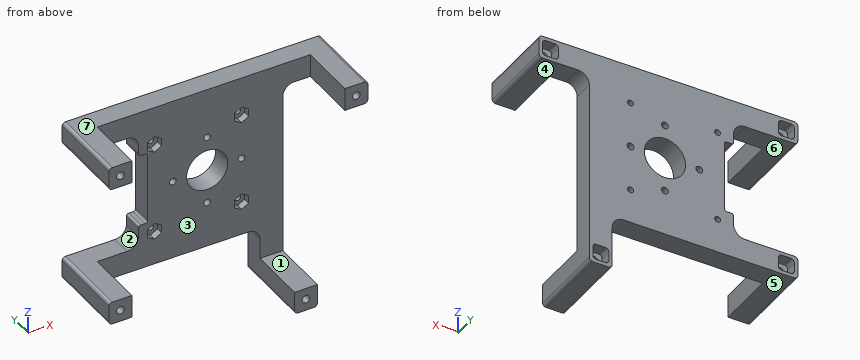
from build123d import *

# Parameters (mm, degrees)
BOSS_EXTRUDE1_DEPTH = 9
CUT_EXTRUDE1_REACH  = 11
SKETCH2_R           = 9
SKETCH2_R_2         = 1.5
CUT_EXTRUDE2_REACH  = 11
SKETCH3_R           = 1.3
SKETCH4_W           = 10
SKETCH4_H           = 10
BOSS_EXTRUDE2_DEPTH = 25.7
SKETCH5_W           = 10
SKETCH5_H           = 10
BOSS_EXTRUDE3_DEPTH = 25.7
SKETCH6_W           = 10
SKETCH6_H           = 10
BOSS_EXTRUDE4_DEPTH = 25.7
SKETCH7_W           = 10
SKETCH7_H           = 10
BOSS_EXTRUDE5_DEPTH = 25.7
SKETCH8_W           = 7
SKETCH8_H           = 7
CUT_EXTRUDE3_DEPTH  = 5
CUT_EXTRUDE4_REACH  = 31.7
SKETCH9_R           = 1.7
FILLET1_R           = 1.5
FILLET2_R           = 5
CUT_EXTRUDE7_DEPTH  = 3
FILLET3_R           = 1


with BuildPart() as part:
    # Sketch1 → Boss-Extrude1 (new body)
    with BuildSketch(Plane(origin=(0, 0, 0), x_dir=(1, 0, 0), z_dir=(0, 1, 0))):
        Polygon((-30, -27), (-30, -17), (-26, -17), (-26, 15), (-30, 15), (-30, 25), (-58, 25), (-58, 35), (23, 35), (23, 59), (33, 59), (33, 35), (33, -27), (55, -27), (55, -37), (33, -37), (-26, -37), (-58, -37), (-58, -27), align=None)
    extrude(amount=BOSS_EXTRUDE1_DEPTH)

    # Sketch2 → Cut-Extrude1 (cut, up to next)
    with BuildSketch(Plane(origin=(0, 9, 0), x_dir=(1, 0, 0), z_dir=(0, 1, 0)), mode=Mode.PRIVATE) as cut_extrude1_sk1:
        Circle(SKETCH2_R)
    cut_extrude1_tool1 = extrude(cut_extrude1_sk1.sketch, amount=-CUT_EXTRUDE1_REACH, mode=Mode.PRIVATE) & part.part
    add(cut_extrude1_tool1.solids().sort_by_distance((0, 9, 0))[0], mode=Mode.SUBTRACT)
    # Sketch2 → Cut-Extrude1 (cut, up to next)
    with BuildSketch(Plane(origin=(0, 9, 0), x_dir=(1, 0, 0), z_dir=(0, 1, 0)), mode=Mode.PRIVATE) as cut_extrude1_sk2:
        with Locations((0, 15)):
            Circle(SKETCH2_R_2)
    cut_extrude1_tool2 = extrude(cut_extrude1_sk2.sketch, amount=-CUT_EXTRUDE1_REACH, mode=Mode.PRIVATE) & part.part
    add(cut_extrude1_tool2.solids().sort_by_distance((0, 9, -15))[0], mode=Mode.SUBTRACT)
    # Sketch2 → Cut-Extrude1 (cut, up to next)
    with BuildSketch(Plane(origin=(0, 9, 0), x_dir=(1, 0, 0), z_dir=(0, 1, 0)), mode=Mode.PRIVATE) as cut_extrude1_sk3:
        with Locations((15, 0)):
            Circle(SKETCH2_R_2)
    cut_extrude1_tool3 = extrude(cut_extrude1_sk3.sketch, amount=-CUT_EXTRUDE1_REACH, mode=Mode.PRIVATE) & part.part
    add(cut_extrude1_tool3.solids().sort_by_distance((15, 9, 0))[0], mode=Mode.SUBTRACT)
    # Sketch2 → Cut-Extrude1 (cut, up to next)
    with BuildSketch(Plane(origin=(0, 9, 0), x_dir=(1, 0, 0), z_dir=(0, 1, 0)), mode=Mode.PRIVATE) as cut_extrude1_sk4:
        with Locations((0, -15)):
            Circle(SKETCH2_R_2)
    cut_extrude1_tool4 = extrude(cut_extrude1_sk4.sketch, amount=-CUT_EXTRUDE1_REACH, mode=Mode.PRIVATE) & part.part
    add(cut_extrude1_tool4.solids().sort_by_distance((0, 9, 15))[0], mode=Mode.SUBTRACT)
    # Sketch2 → Cut-Extrude1 (cut, up to next)
    with BuildSketch(Plane(origin=(0, 9, 0), x_dir=(1, 0, 0), z_dir=(0, 1, 0)), mode=Mode.PRIVATE) as cut_extrude1_sk5:
        with Locations((-15, 0)):
            Circle(SKETCH2_R_2)
    cut_extrude1_tool5 = extrude(cut_extrude1_sk5.sketch, amount=-CUT_EXTRUDE1_REACH, mode=Mode.PRIVATE) & part.part
    add(cut_extrude1_tool5.solids().sort_by_distance((-15, 9, 0))[0], mode=Mode.SUBTRACT)

    # Sketch3 → Cut-Extrude2 (cut, up to next)
    with BuildSketch(Plane(origin=(0, 9, 0), x_dir=(1, 0, 0), z_dir=(0, 1, 0)), mode=Mode.PRIVATE) as cut_extrude2_sk1:
        with Locations((-23, 20)):
            Circle(SKETCH3_R)
    cut_extrude2_tool1 = extrude(cut_extrude2_sk1.sketch, amount=-CUT_EXTRUDE2_REACH, mode=Mode.PRIVATE) & part.part
    add(cut_extrude2_tool1.solids().sort_by_distance((-23, 9, -20))[0], mode=Mode.SUBTRACT)
    # Sketch3 → Cut-Extrude2 (cut, up to next)
    with BuildSketch(Plane(origin=(0, 9, 0), x_dir=(1, 0, 0), z_dir=(0, 1, 0)), mode=Mode.PRIVATE) as cut_extrude2_sk2:
        with Locations((-23, -20)):
            Circle(SKETCH3_R)
    cut_extrude2_tool2 = extrude(cut_extrude2_sk2.sketch, amount=-CUT_EXTRUDE2_REACH, mode=Mode.PRIVATE) & part.part
    add(cut_extrude2_tool2.solids().sort_by_distance((-23, 9, 20))[0], mode=Mode.SUBTRACT)
    # Sketch3 → Cut-Extrude2 (cut, up to next)
    with BuildSketch(Plane(origin=(0, 9, 0), x_dir=(1, 0, 0), z_dir=(0, 1, 0)), mode=Mode.PRIVATE) as cut_extrude2_sk3:
        with Locations((15, 20)):
            Circle(SKETCH3_R)
    cut_extrude2_tool3 = extrude(cut_extrude2_sk3.sketch, amount=-CUT_EXTRUDE2_REACH, mode=Mode.PRIVATE) & part.part
    add(cut_extrude2_tool3.solids().sort_by_distance((15, 9, -20))[0], mode=Mode.SUBTRACT)
    # Sketch3 → Cut-Extrude2 (cut, up to next)
    with BuildSketch(Plane(origin=(0, 9, 0), x_dir=(1, 0, 0), z_dir=(0, 1, 0)), mode=Mode.PRIVATE) as cut_extrude2_sk4:
        with Locations((15, -20)):
            Circle(SKETCH3_R)
    cut_extrude2_tool4 = extrude(cut_extrude2_sk4.sketch, amount=-CUT_EXTRUDE2_REACH, mode=Mode.PRIVATE) & part.part
    add(cut_extrude2_tool4.solids().sort_by_distance((15, 9, 20))[0], mode=Mode.SUBTRACT)

    # Sketch4 → Boss-Extrude2 (add)
    with BuildSketch(Plane.XZ):
        with Locations((-53, -30)):
            Rectangle(SKETCH4_W, SKETCH4_H)
    extrude(amount=BOSS_EXTRUDE2_DEPTH)

    # Sketch5 → Boss-Extrude3 (add)
    with BuildSketch(Plane.XZ):
        with Locations((-53, 32)):
            Rectangle(SKETCH5_W, SKETCH5_H)
    extrude(amount=BOSS_EXTRUDE3_DEPTH)

    # Sketch6 → Boss-Extrude4 (add)
    with BuildSketch(Plane.XZ):
        with Locations((28, -54)):
            Rectangle(SKETCH6_W, SKETCH6_H)
    extrude(amount=BOSS_EXTRUDE4_DEPTH)

    # Sketch7 → Boss-Extrude5 (add)
    with BuildSketch(Plane.XZ):
        with Locations((50, 32)):
            Rectangle(SKETCH7_W, SKETCH7_H)
    extrude(amount=BOSS_EXTRUDE5_DEPTH)

    # Sketch8 → Cut-Extrude3 (cut)
    with BuildSketch(Plane(origin=(0, 9, 0), x_dir=(1, 0, 0), z_dir=(0, 1, 0))):
        with Locations((-53, 30)):
            Rectangle(SKETCH8_W, SKETCH8_H)
        with Locations((-53, -32)):
            Rectangle(SKETCH8_W, SKETCH8_H)
        with Locations((50, -32)):
            Rectangle(SKETCH8_W, SKETCH8_H)
        with Locations((28, 54)):
            Rectangle(SKETCH8_W, SKETCH8_H)
    extrude(amount=-CUT_EXTRUDE3_DEPTH, mode=Mode.SUBTRACT)

    # Sketch9 → Cut-Extrude4 (cut, up to next)
    with BuildSketch(Plane(origin=(0, 4, 0), x_dir=(1, 0, 0), z_dir=(0, 1, 0)), mode=Mode.PRIVATE) as cut_extrude4_sk1:
        with Locations((-53, 30)):
            Circle(SKETCH9_R)
    cut_extrude4_tool1 = extrude(cut_extrude4_sk1.sketch, amount=-CUT_EXTRUDE4_REACH, mode=Mode.PRIVATE) & part.part
    add(cut_extrude4_tool1.solids().sort_by_distance((-53, 4, -30))[0], mode=Mode.SUBTRACT)
    # Sketch9 → Cut-Extrude4 (cut, up to next)
    with BuildSketch(Plane(origin=(0, 4, 0), x_dir=(1, 0, 0), z_dir=(0, 1, 0)), mode=Mode.PRIVATE) as cut_extrude4_sk2:
        with Locations((28, 54)):
            Circle(SKETCH9_R)
    cut_extrude4_tool2 = extrude(cut_extrude4_sk2.sketch, amount=-CUT_EXTRUDE4_REACH, mode=Mode.PRIVATE) & part.part
    add(cut_extrude4_tool2.solids().sort_by_distance((28, 4, -54))[0], mode=Mode.SUBTRACT)
    # Sketch9 → Cut-Extrude4 (cut, up to next)
    with BuildSketch(Plane(origin=(0, 4, 0), x_dir=(1, 0, 0), z_dir=(0, 1, 0)), mode=Mode.PRIVATE) as cut_extrude4_sk3:
        with Locations((50, -32)):
            Circle(SKETCH9_R)
    cut_extrude4_tool3 = extrude(cut_extrude4_sk3.sketch, amount=-CUT_EXTRUDE4_REACH, mode=Mode.PRIVATE) & part.part
    add(cut_extrude4_tool3.solids().sort_by_distance((50, 4, 32))[0], mode=Mode.SUBTRACT)
    # Sketch9 → Cut-Extrude4 (cut, up to next)
    with BuildSketch(Plane(origin=(0, 4, 0), x_dir=(1, 0, 0), z_dir=(0, 1, 0)), mode=Mode.PRIVATE) as cut_extrude4_sk4:
        with Locations((-53, -32)):
            Circle(SKETCH9_R)
    cut_extrude4_tool4 = extrude(cut_extrude4_sk4.sketch, amount=-CUT_EXTRUDE4_REACH, mode=Mode.PRIVATE) & part.part
    add(cut_extrude4_tool4.solids().sort_by_distance((-53, 4, 32))[0], mode=Mode.SUBTRACT)

    # Fillet1
    fillet1_edges = [part.edges().sort_by_distance(p)[0] for p in [
        (24.5, 6.5, -57.5),
        (24.5, 6.5, -50.5),
        (31.5, 6.5, -50.5),
        (31.5, 6.5, -57.5),
        (46.5, 6.5, 28.5),
        (46.5, 6.5, 35.5),
        (53.5, 6.5, 35.5),
        (53.5, 6.5, 28.5),
        (-56.5, 6.5, 28.5),
        (-56.5, 6.5, 35.5),
        (-49.5, 6.5, 35.5),
        (-49.5, 6.5, 28.5),
        (-49.5, 6.5, -26.5),
        (-49.5, 6.5, -33.5),
        (-56.5, 6.5, -33.5),
        (-56.5, 6.5, -26.5),
        (-58, -8.35, -35),
        (23, -8.35, -59),
        (33, -8.35, -59),
        (55, -8.35, 27),
        (55, -8.35, 37),
        (-58, -8.35, 37),
        (-58, -8.35, 27),
        (-58, -8.35, -25),
    ]]
    fillet(fillet1_edges, radius=FILLET1_R)

    # Fillet2
    fillet2_edges = [part.edges().sort_by_distance(p)[0] for p in [
        (23, 4.5, -35),
        (33, 4.5, 27),
        (-30, 4.5, 27),
        (-30, 4.5, -25),
    ]]
    fillet(fillet2_edges, radius=FILLET2_R)

    # Sketch12 → Cut-Extrude7 (cut)
    with BuildSketch(Plane.XZ):
        Polygon((-19.9, 18.210214166), (-19.9, 21.789785834), (-23, 23.579571669), (-26.1, 21.789785834), (-26.1, 18.210214166), (-23, 16.420428331), align=None)
        Polygon((18.1, 21.789785834), (15, 23.579571669), (11.9, 21.789785834), (11.9, 18.210214166), (15, 16.420428331), (18.1, 18.210214166), align=None)
        Polygon((18.1, -18.210214166), (15, -16.420428331), (11.9, -18.210214166), (11.9, -21.789785834), (15, -23.579571669), (18.1, -21.789785834), align=None)
        Polygon((-19.9, -18.210214166), (-23, -16.420428331), (-26.1, -18.210214166), (-26.1, -21.789785834), (-23, -23.579571669), (-19.9, -21.789785834), align=None)
    extrude(amount=-CUT_EXTRUDE7_DEPTH, mode=Mode.SUBTRACT)

    # Fillet3
    fillet3_edges = [part.edges().sort_by_distance(p)[0] for p in [
        (-30, 4.5, 17),
        (-26, 4.5, 17),
        (-26, 4.5, -15),
        (-30, 4.5, -15),
    ]]
    fillet(fillet3_edges, radius=FILLET3_R)


solid = part.part
Source: CAD feature listing. Evaluate the final solid. Frame: model axes, mm. Face numbers are marked on the shaded views. A direction names the side the tool comes from. Coordinates: 2 decimals unless noted, no trailing zeros. Write each loop counter-clockwise with the first axis right and the second up, starting at its lowest first coordinate (ties: lowest second). Pieces come first, ordered by that corner, then holes. Notation, with made-up numbers: M -14,75 L 39,75 A15 cw 39,101 Z; hole C -20,-38 d9. An arc over 180 degrees is marked long. Use a Markdown table: item, result.
1) Section A-A, the plane x = -53. Output: boundary loops of the cut face in (y, z).
Conclusion:
| item | result |
|---|---|
| outline | M -25.7,-35 L 9,-35 L 9,-33.5 L 4,-33.5 L 4,-31.7 L -25.7,-31.7 Z; M -25.7,-28.3 L 4,-28.3 L 4,-26.5 L 9,-26.5 L 9,-25 L -25.7,-25 Z; M -25.7,27 L 9,27 L 9,28.5 L 4,28.5 L 4,30.3 L -25.7,30.3 Z; M -25.7,33.7 L 4,33.7 L 4,35.5 L 9,35.5 L 9,37 L -25.7,37 Z |
2) Section C-C, the plane y = -9. Output: boundary loops of the cut face in (x, z), then the cut area to 3 significant figures.
Conclusion:
| item | result |
|---|---|
| outline | M -58,-33.5 A1.5 ccw -56.5,-35 L -48,-35 L -48,-25 L -56.5,-25 A1.5 ccw -58,-26.5 Z; M -58,28.5 A1.5 ccw -56.5,27 L -48,27 L -48,37 L -56.5,37 A1.5 ccw -58,35.5 Z; M 23,-57.5 A1.5 ccw 24.5,-59 L 31.5,-59 A1.5 ccw 33,-57.5 L 33,-49 L 23,-49 Z; M 45,27 L 53.5,27 A1.5 ccw 55,28.5 L 55,35.5 A1.5 ccw 53.5,37 L 45,37 Z; hole C -53,-30 d3.4; hole C -53,32 d3.4; hole C 28,-54 d3.4; hole C 50,32 d3.4 |
| area | 360 mm^2 |
3) Reachability of the marked faces 1, 2, 3 and 4 from +Z, -Z, +X, -X, +Y, -Y: full face, straight path, thin tool, end or side. Return the list, or none.
Conclusion:
| item | result |
|---|---|
| face 1 | +Z, +X, -X, -Y |
| face 2 | -X, +Y, -Y |
| face 3 | +Z, -Y |
| face 4 | -Z, +X, +Y, -Y |
4) Section D-D, the plane x = -36.5. Output: boundary loops of the cut face in (y, z).
Conclusion:
| item | result |
|---|---|
| outline | M 0,-35 L 9,-35 L 9,-25 L 0,-25 Z; M 0,27 L 9,27 L 9,37 L 0,37 Z |
5) Section B-B, the plane z = -30. Output: boundary loops of the cut face in (x, y), then the cut area to 3 significant figures.
Conclusion:
| item | result |
|---|---|
| outline | M -58,-25.7 L -54.7,-25.7 L -54.7,4 L -56.5,4 L -56.5,9 L -58,9 Z; M -51.3,-25.7 L -48,-25.7 L -48,0 L 33,0 L 33,9 L -49.5,9 L -49.5,4 L -51.3,4 Z |
| area | 940 mm^2 |
6) Mould query, pull axis Z, two halves, no side actions, for the marked faces 5, 6 and 7. Classes: pulls with the +Z half, pulls with the -Z half, needs draft (parallel to the pull), parting line crosses it, or undercut.
Conclusion:
| item | result |
|---|---|
| face 5 | pulls with the -Z half |
| face 6 | undercut |
| face 7 | pulls with the +Z half |
7) Ray query, L1, parallel to Z at x = 0, y = 5; L2, parallel to Z at x = -23, y = 4; L3, parallel to X at y = 4.75, z = 0. Return the intervals inside material, ascending.
Conclusion:
| item | result |
|---|---|
| L1 | z = -35 to -16.5, -13.5 to -9, 9 to 13.5, 16.5 to 37 |
| L2 | z = -35 to -21.3, -18.7 to 18.7, 21.3 to 37 |
| L3 | x = -26 to -16.5, -13.5 to -9, 9 to 13.5, 16.5 to 33 |
8) First-contact query: pin 1 Ø3 at (x, z) = (-24, -21) entering from -Y; pin 2 Ø4.5 at (y, z) = (6.5, -53.5) entering from -X; pin 3 Ø1.5 at (y, z) = (1, -20) entering from +X; pin 4 Ø2.5 at (x, z) = (-23, -20) entering from -Y. Flat tips, straight axial feed; report the tip coordinate or a pass-through.
Conclusion:
| item | result |
|---|---|
| pin 1 | stops at y = 3 |
| pin 2 | stops at x = 23 |
| pin 3 | stops at x = 33 |
| pin 4 | passes through |
